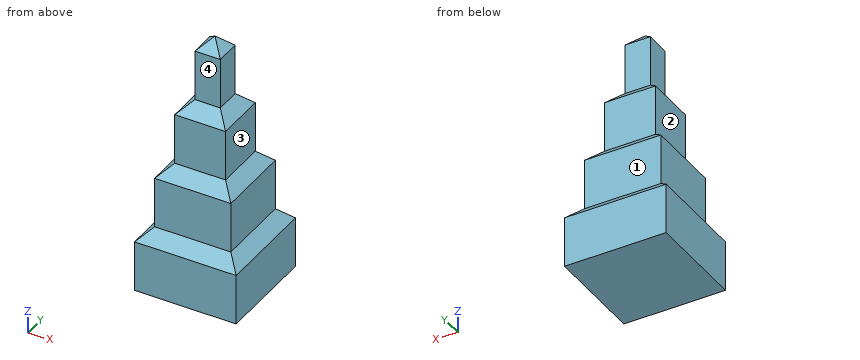
```python
from build123d import *

# Parameters (mm, degrees)
F0_W     = 8
F0_H     = 8
F0_W_2   = 6
F0_H_2   = 6
F1_DEPTH = 5
F0_W_3   = 4
F0_H_3   = 4
F2_DEPTH = 10
F0_W_4   = 2
F0_H_4   = 2
F3_DEPTH = 15
F4_DEPTH = 20
F5_SIZE  = 0.99999


# Not quite as in the source:
# - a fillet or chamfer is up to 0.001 mm smaller than in the source, because OpenCascade refuses the exact size


with BuildPart() as f1:
    # F0 (on Top) → F1 (new body)
    with BuildSketch(Plane.XY):
        Rectangle(F0_W, F0_H)
        Rectangle(F0_W_2, F0_H_2, mode=Mode.SUBTRACT)
    extrude(amount=F1_DEPTH)

    # F0 (on Top) → F2 (join)
    with BuildSketch(Plane.XY):
        Rectangle(F0_W_2, F0_H_2)
        Rectangle(F0_W_3, F0_H_3, mode=Mode.SUBTRACT)
    extrude(amount=F2_DEPTH)

    # F0 (on Top) → F3 (join)
    with BuildSketch(Plane.XY):
        Rectangle(F0_W_3, F0_H_3)
        Rectangle(F0_W_4, F0_H_4, mode=Mode.SUBTRACT)
    extrude(amount=F3_DEPTH)

    # F0 (on Top) → F4 (join)
    with BuildSketch(Plane.XY):
        Rectangle(F0_W_4, F0_H_4)
    extrude(amount=F4_DEPTH)

    # F5 (size 1 in the source; OpenCascade refuses exactly that, so slightly less here)
    f5_edges = [f1.edges().sort_by_distance(p)[0] for p in [
        (0, -4, 5),
        (4, 0, 5),
        (0, 4, 5),
        (-4, 0, 5),
        (0, -3, 10),
        (3, 0, 10),
        (-3, 0, 10),
        (0, 3, 10),
        (2, 0, 15),
        (0, -2, 15),
        (-2, 0, 15),
        (0, 2, 15),
        (1, 0, 20),
        (0, -1, 20),
        (-1, 0, 20),
        (0, 1, 20),
    ]]
    chamfer(f5_edges, length=F5_SIZE)


solid = f1.part
```
Can you work these out from the model? Positions are in its coordinate system, mm. Face numbers are marked on the shaded views. A direction names the side the tool comes from. Round coordinates to 2 decimals unless told otherwise and drop trailing zeros. Loops run counter-clockwise (first coordinate to the right, second up) from the corner with the lowest first, then second, coordinate; pieces in that order, holes last. Notation, with made-up numbers: (-24.75, 68.5) -> (-20.75, 68.5) arc R15 ccw to (-20.75, 88.5) -> close; hole circle Ø2 at (69.5, -27). An arc over 180 degrees is marked (long way). Answer in a Markdown table with one row per item.
Item 1: Will these pins go through, and if not, where does the flat tip stop? P1, Ø4, axis at x = 1.5, y = -2, coming from the +Z side; P2, Ø2, axis at y = 0.5, z = 18, coming from the -X side; P3, Ø1.2, axis at x = 1, z = 7.5, coming from the -Y side; P4, Ø1.5, axis at x = 1, y = 2, coming from the -Z side.
Answer block:
| item | result |
|---|---|
| P1 | z = 19.64 |
| P2 | x = -1 |
| P3 | y = -3 |
| P4 | z = 0 |
Item 2: Suppose I cut it at D-D, the plane y = 3.75. List the corners of the cut face in (x, z) for me, plus the area to 3 significant figures.
Answer block:
| item | result |
|---|---|
| outline | (-4, 0) -> (4, 0) -> (4, 4) -> (3.75, 4.25) -> (-3.75, 4.25) -> (-4, 4) -> close |
| area | 33.9 mm² |
Item 3: Suppose I cut it at C-C, the plane z = 8.75. List the corners of the cut face in (x, y) for me.
Answer block:
| item | result |
|---|---|
| outline | (-3, -3) -> (3, -3) -> (3, 3) -> (-3, 3) -> close |
Item 4: If I drill on probe 1 along X at (y, z) = (0.5, 16.5); probe 2 along X at (y, z) = (1.5, 13); probe 3 along Y at (x, z) = (2.5, 5.75), over which ranges is the centre line in solid material (lowest first)?
Answer block:
| item | result |
|---|---|
| probe 1 | -1 to 1 |
| probe 2 | -2 to 2 |
| probe 3 | -3 to 3 |
Item 5: On a 3-axis mill with a long thin cutter (end or side, diameter ignored), from which of +Z, -Z, +X, -X, +Y, -Y can I reach the whole of each face in a straight line? I mean the marked faces 1, 2, 3 and 4. Say none if no direction works.
Answer block:
| item | result |
|---|---|
| face 1 | +Z, +X, -X, +Y |
| face 2 | +Z, -X, +Y, -Y |
| face 3 | +Z, +X, +Y, -Y |
| face 4 | +Z, +X, -X, -Y |
